Could you check a few things on this drawing? It's one solid part, dimensions in mm from its lowest x, y, z. A direction names the side the tool comes from. Give positions to 0.01 mm unless a question says otherwise; leave off trailing zeros. Order: outer loops, then holes, each group sorted by start corner. A loop starts at its lowest first (then second) coordinate and runs counter-clockwise, first axis right, second up. Notation, with made-up numbers: (49, 5) - (62, 5) arc R30 ccw to (62, 27) - close; hole circle Ø10 at (6, 30.5). An arc over 180 degrees is marked (long way). One line per question, with ' | ' between items. Start each with the question number.
1. I need wall thicknesses on probe 1 along Y at (x, z) = (13.5, 2); probe 2 along X at (y, z) = (45.5, 9.5) (1 decimal); probe 3 along X at (y, z) = (49.5, 11). Which ranges of each line are inside material? Lowest first, please. Write a range as from..to.
2. Imagine slicing it at B-B (x = 35). Please give me the cut outline in (y, z) (1 decimal), and give its area (3 significant figures).
3. Imagine slicing it at C-C (y = 10). Please give me the cut outline in (x, z), and give its area (3 significant figures).
4. For P1, Ø3, axis at x = 31, z = 20.5, coming from the -Y side; P2, Ø6, axis at x = 9.5, y = 47.5, coming from the -Z side; P3, Ø5, axis at y = 34, z = 10.5, coming from the -X side; P4, Ø2, axis at x = 16, y = 68, coming from the -Z side, each with a flat end and sliding along its axis, tell me the tip position at first contact or that it passes through.
5. Which directions (+Z, -Z, +X, -X, +Y, -Y) give clear straight access to the entire face, cutting with the end or side of a thin tool? Please do the marked faces 1 and 2.
6. Imagine slicing it at A-A (y = 67). Please give me the cut outline in (x, z) (1 decimal).
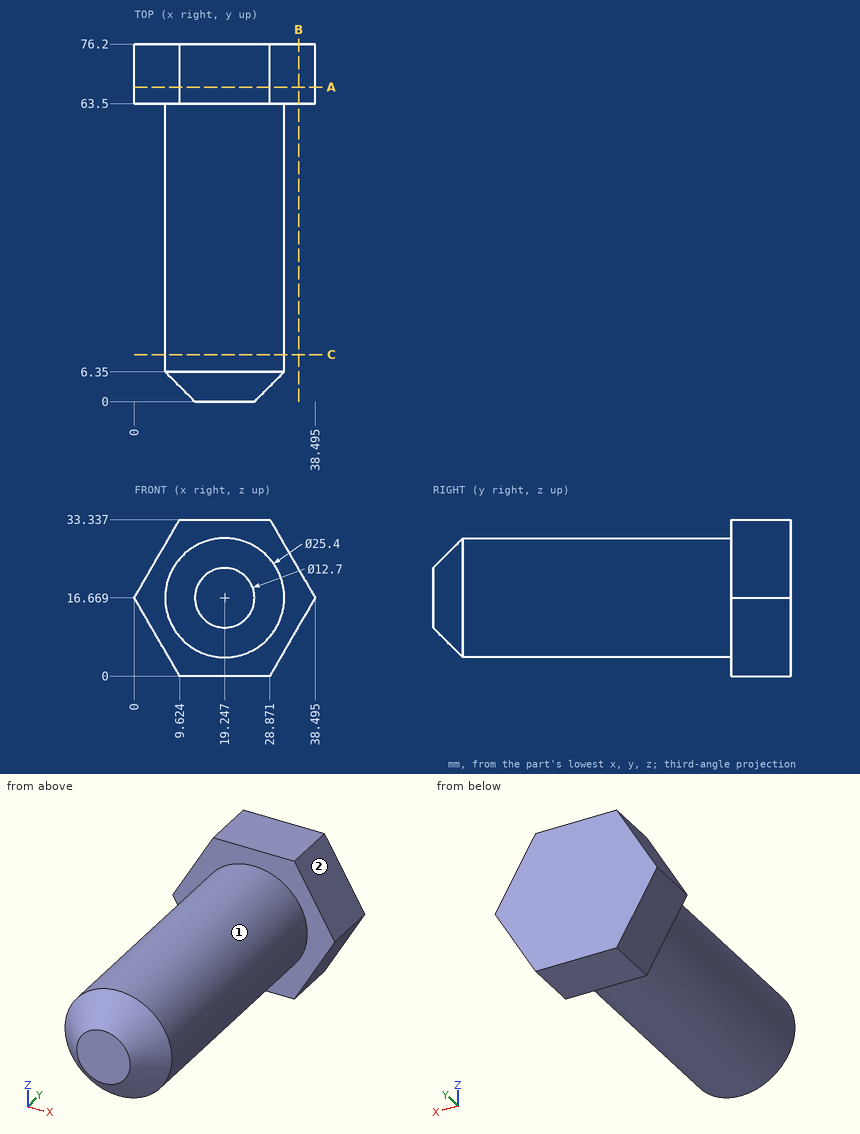
Results found:
1) probe 1: y = 63.5..76.2 | probe 2: x = 8.8..29.7 | probe 3: x = 7.88..30.61
2) outline: (63.5, 10.6) - (76.2, 10.6) - (76.2, 22.7) - (63.5, 22.7) - close | area: 154 mm2
3) outline: circle Ø25.4 at (19.25, 16.67) | area: 507 mm2
4) P1: stops at y = 4.51 | P2: stops at z = 5.91 | P3: stops at x = 7.09 | P4: stops at z = 0
5) face 1: -Y | face 2: +Z, +X, +Y, -Y
6) outline: (0, 16.7) - (9.6, 0) - (28.9, 0) - (38.5, 16.7) - (28.9, 33.3) - (9.6, 33.3) - close
